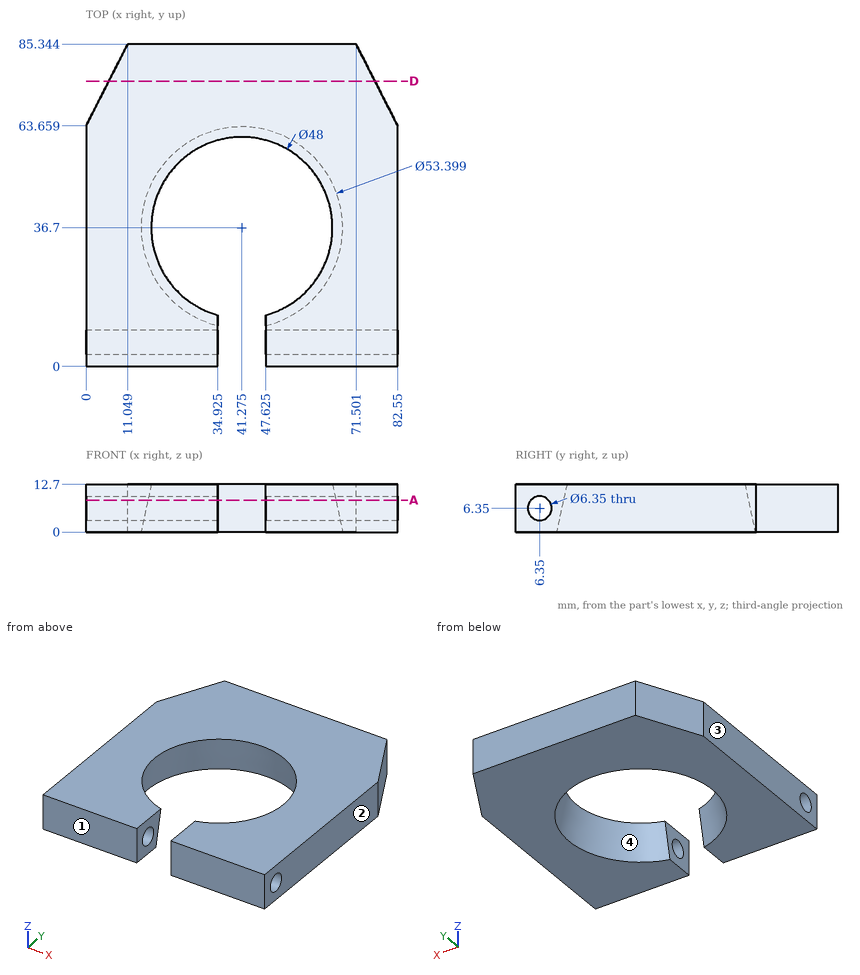
Could you check a few things on this drawing? It's one solid part, dimensions in mm from its lowest x, y, z. Give positions to 0.01 mm unless a question says otherwise; leave off trailing zeros. Order: outer loops, then holes, each group sorted by start corner. A loop starts at its lowest first (then second) coordinate and runs counter-clockwise, first axis right, second up. Notation, with made-up numbers: (79.5, -26.5) -> (123.5, -26.5) arc R12 cw to (123.5, -8.5) -> close; hole circle Ø2 at (3, 79). An arc over 180 degrees is marked (long way). Answer in a Markdown table with one row per item. Add a question column.
Item 1: Please list where these lines run through material, in increasing order: probe 1 along X at (y, z) = (9, 11.75) (3 decimals); probe 2 along Z at (x, y) = (70, 6); probe 3 along Y at (x, z) = (56.5, 9).
Item 2: We'd pull the mould along X, two halves only. Please class the marked faces 1, 2, 3 and 4: pulls with the +X half, pulls with the -X half, needs draft (parallel to the pull), parting line crosses it, or undercut.
Item 3: Imagine slicing it at D-D (y = 75.5). List the corners of the cut face in (x, z) for me.
Item 4: I'm going to push a flat-ended pin straight in: P1, Ø5, axis at x = 43.5, z = 9, coming from the -Y side. Where does the tip first touch, or does it pass through?
Item 5: Imagine slicing it at A-A (z = 8.5). Count the separate pieces of the cut face and the enclosed holes in it, and give its area (3 significant figures).
Result:
| question | item | result |
|---|---|---|
| 1 | probe 1 | 0 to 34.925, 47.625 to 82.55 |
| 1 | probe 2 | 0 to 3.19, 9.51 to 12.7 |
| 1 | probe 3 | 0 to 4.6, 8.1 to 17.14, 56.26 to 85.34 |
| 2 | face 1 | needs draft |
| 2 | face 2 | pulls with the +X half |
| 2 | face 3 | pulls with the -X half |
| 2 | face 4 | undercut |
| 3 | outline | (6.03, 0) -> (76.52, 0) -> (76.52, 12.7) -> (6.03, 12.7) -> close |
| 4 | P1 | y = 60.77 |
| 5 | separate pieces | 3 |
| 5 | enclosed holes | 0 |
| 5 | area | 4,380 mm2 |
